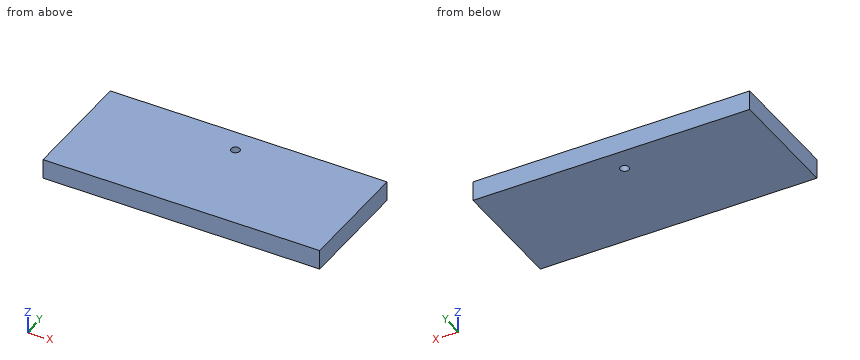
from build123d import *

# Parameters (mm, degrees)
SKETCH1_W               = 700
SKETCH1_H               = 300
BOSS_EXTRUDE1_DEPTH     = 25
SKETCH2_R               = 11
CUT_EXTRUDE1_DEPTH      = 26
CUT_EXTRUDE1_DEPTH_BACK = 26


with BuildPart() as part:
    # Sketch1 → Boss-Extrude1 (new body, symmetric)
    with BuildSketch(Plane.XY):
        with Locations((0, 150)):
            Rectangle(SKETCH1_W, SKETCH1_H)
    extrude(amount=BOSS_EXTRUDE1_DEPTH, both=True)

    # Sketch2 → Cut-Extrude1 (cut, two sides)
    with BuildSketch(Plane.XY) as cut_extrude1_sk:
        with Locations((0, 241)):
            Circle(SKETCH2_R)
    extrude(amount=CUT_EXTRUDE1_DEPTH, mode=Mode.SUBTRACT)
    extrude(cut_extrude1_sk.sketch, amount=-CUT_EXTRUDE1_DEPTH_BACK, mode=Mode.SUBTRACT)


solid = part.part
The model under review builds one solid part; all positions refer to its coordinate system, in mm. Round coordinates to 2 decimals unless told otherwise and drop trailing zeros. Write each loop counter-clockwise with the first axis right and the second up, starting at its lowest first coordinate (ties: lowest second). Pieces come first, ordered by that corner, then holes. Notation, with made-up numbers: (63, -10.5) -> (90, -10.5) arc R22 ccw to (90, 0.5) -> close; hole circle Ø3 at (33.25, 59.25). An arc over 180 degrees is marked (long way). Answer as a JSON object with one key per item and string values.
1. We need section A-A on x = 0. State the section outline as (y, z) points.
Results found:
{"outline": "(0, -25) -> (230, -25) -> (230, 25) -> (0, 25) -> close; (252, -25) -> (300, -25) -> (300, 25) -> (252, 25) -> close"}
2. We need section B-B on y = 241. State the section outline as (x, z) points.
Results found:
{"outline": "(-350, -25) -> (-11, -25) -> (-11, 25) -> (-350, 25) -> close; (11, -25) -> (350, -25) -> (350, 25) -> (11, 25) -> close"}
3. To check wall thickness, follow line 1 along Y through (x, z) = (0, -1); line 2 along X through (y, z) = (241, 9.5); line 3 along X through (y, z) = (238, -5.5). State the ranges of each line that lie inside material, in increasing order.
Results found:
{"line 1": "y = 0 to 230, 252 to 300", "line 2": "x = -350 to -11, 11 to 350", "line 3": "x = -350 to -10.58, 10.58 to 350"}
